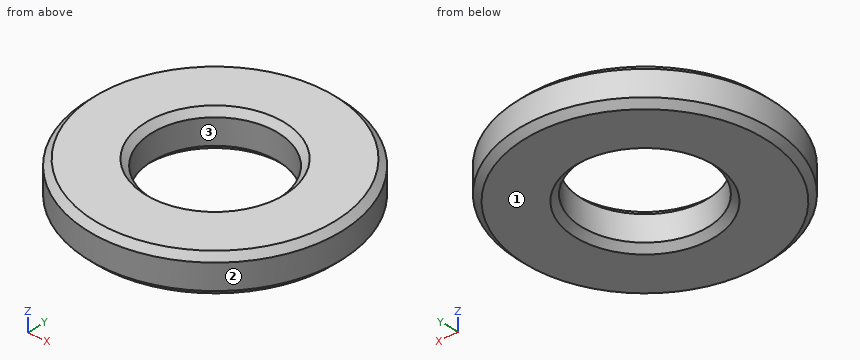
Autodesk Inventor part; units mm, degrees
ref_plane "YZ Plane" through (0, 0, 0) normal (1, 0, 0) x (0, 1, 0)
ref_plane "XZ Plane" through (0, 0, 0) normal (0, 1, 0) x (-1, 0, 0)
ref_plane "XY Plane" through (0, 0, 0) normal (0, 0, 1) x (1, 0, 0)
sketch "スケッチ1" plane through (0, 0, 0) normal (0, 0, 1) x (1, 0, 0)
  circle A0 centre (0, 0) radius 10
  dimension "d0" = 20
extrude "押し出し1" add sketch "スケッチ1" along normal blind 3
sketch "スケッチ2" plane through (0, 0, 3) normal (0, 0, 1) x (1, 0, 0)
  circle A0 centre (0, 0) radius 10
hole "穴1" at (0, 0, 3) direction (0, 0, -1) diameter 10 end through all
chamfer "面取り1" distance 0.5 angle 45 4 edges at (-10, 0, 3) (-10, 0, 0) (0, 5, 3) (0, 5, 0)
properties part number "WSSM20-10-3" material "MISUMI"
Could you check a few things on this model? Use its own coordinates, in mm. Face numbers are marked on the shaded views. Coordinates: 2 decimals unless noted, no trailing zeros. Write each loop counter-clockwise with the first axis right and the second up, starting at its lowest first coordinate (ties: lowest second). Pieces come first, ordered by that corner, then holes. Notation, with made-up numbers: (-39.5, 52) - (13.5, 52) arc R15 cw to (13.5, 80) - close; hole circle Ø6 at (40, 31). An arc over 180 degrees is marked (long way). Use a Markdown table: item, result.
Q1. Imagine slicing it at D-D (z = 2.75). List the corners of the cut face in (x, y) for me.
Geometry check:
| item | result |
|---|---|
| outline | circle Ø19.5 at (0, 0); hole circle Ø10.5 at (0, 0) |
Q2. Imagine slicing it at C-C (z = 1.1). List the corners of the cut face in (x, y) for me, and give its area (3 significant figures).
Geometry check:
| item | result |
|---|---|
| outline | circle Ø20 at (0, 0); hole circle Ø10 at (0, 0) |
| area | 236 mm2 |
Q3. I'm going to push a flat-ended pin straight in: pin 1 Ø1 at (y, z) = (7, 2) entering from +X. Where does the tip first touch, or does it pass through?
Geometry check:
| item | result |
|---|---|
| pin 1 | stops at x = 7.6 |
Q4. Please list where these lines run through material, in increasing order: L1, parallel to Y at x = 0, z = 1.05; L2, parallel to Y at x = 4.5, z = 0.6; L3, parallel to X at y = -2.5, z = 0.45.
Geometry check:
| item | result |
|---|---|
| L1 | y = -10 to -5, 5 to 10 |
| L2 | y = -8.93 to -2.18, 2.18 to 8.93 |
| L3 | x = -9.63 to -4.39, 4.39 to 9.63 |
Q5. Imagine slicing it at A-A (y = 0). List the corners of the cut face in (x, z) for me, and give its area (3 significant figures).
Geometry check:
| item | result |
|---|---|
| outline | (-10, 0.5) - (-9.5, 0) - (-5.5, 0) - (-5, 0.5) - (-5, 2.5) - (-5.5, 3) - (-9.5, 3) - (-10, 2.5) - close; (5, 0.5) - (5.5, 0) - (9.5, 0) - (10, 0.5) - (10, 2.5) - (9.5, 3) - (5.5, 3) - (5, 2.5) - close |
| area | 29.0 mm2 |
Q6. Thinking about a two-plate mould opening in Y: for the marked faces 1, 2 and 3, which applies, +Y half, -Y half, draft (parallel to the pull), parting line (faces both ways), or undercut?
Geometry check:
| item | result |
|---|---|
| face 1 | draft |
| face 2 | parting line |
| face 3 | undercut |
